Can you work these out from the drawing? Everything is in mm from the part's minimum corner. A direction names the side the tool comes from. Round coordinates to 2 decimals unless told otherwise and drop trailing zeros. Order: outer loops, then holes, each group sorted by start corner. A loop starts at its lowest first (then second) coordinate and runs counter-clockwise, first axis right, second up. Notation, with made-up numbers: (23, 17.5) -> (61, 17.5) arc R31 cw to (61, 51.5) -> close; hole circle Ø8 at (84, 60.25). An arc over 180 degrees is marked (long way). One line per item, written item: value.
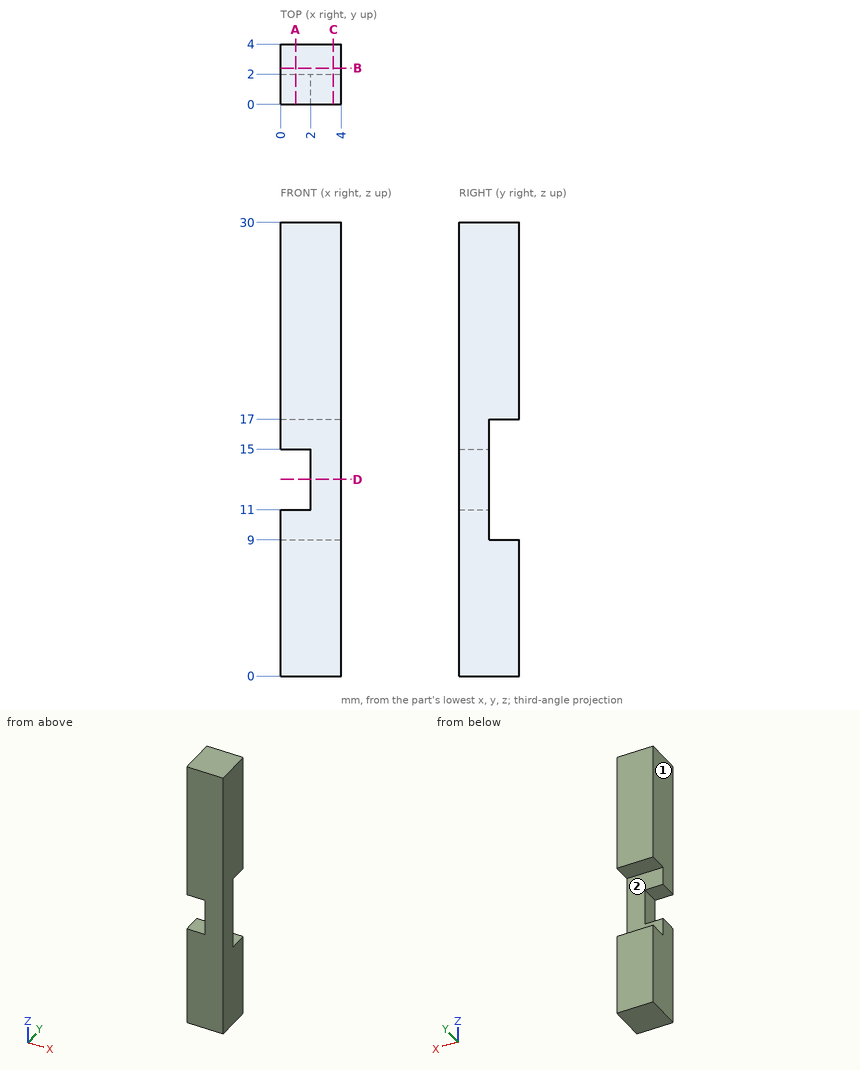
Q1. For P1, Ø2, axis at x = 2.5, z = 12.5, coming from the +Y side; P2, Ø1.6, axis at y = 1, z = 12.5, coming from the -X side, each with a flat end and sliding along its axis, tell me the tip position at first contact or that it passes through.
Answers:
P1: y = 2
P2: x = 2
Q2. I want a section at B-B on y = 2.4. Write out the boundary of the cut face in (x, z), then the cut area to 3 significant figures.
Answers:
outline: (0, 0) -> (4, 0) -> (4, 9) -> (0, 9) -> close; (0, 17) -> (4, 17) -> (4, 30) -> (0, 30) -> close
area: 88.0 mm2
Q3. I need wall thicknesses on line 1 along Z through (x, y) = (0.55, 3.45); line 2 along Z through (x, y) = (0.65, 0.85); line 3 along Y through (x, z) = (2.85, 13). Which ranges of each line are inside material? Lowest first, please.
Answers:
line 1: 0 to 9, 17 to 30
line 2: 0 to 11, 15 to 30
line 3: 0 to 2
Q4. I want a section at C-C on x = 3.5. Write out the boundary of the cut face in (y, z), then the cut area to 3 significant figures.
Answers:
outline: (0, 0) -> (4, 0) -> (4, 9) -> (2, 9) -> (2, 17) -> (4, 17) -> (4, 30) -> (0, 30) -> close
area: 104 mm2
Q5. Which directions (+Z, -Z, +X, -X, +Y, -Y) give clear straight access to the entire face, cutting with the end or side of a thin tool? Please do the marked faces 1 and 2.
Answers:
face 1: +Z, -Z, -X, +Y, -Y
face 2: +X, -X, +Y
Q6. I want a section at A-A on x = 1. Write out the boundary of the cut face in (y, z), then the cut area to 3 significant figures.
Answers:
outline: (0, 0) -> (4, 0) -> (4, 9) -> (2, 9) -> (2, 11) -> (0, 11) -> close; (0, 15) -> (2, 15) -> (2, 17) -> (4, 17) -> (4, 30) -> (0, 30) -> close
area: 96.0 mm2
Q7. I want a section at D-D on z = 13. Write out the boundary of the cut face in (x, y).
Answers:
outline: (2, 0) -> (4, 0) -> (4, 2) -> (2, 2) -> close
